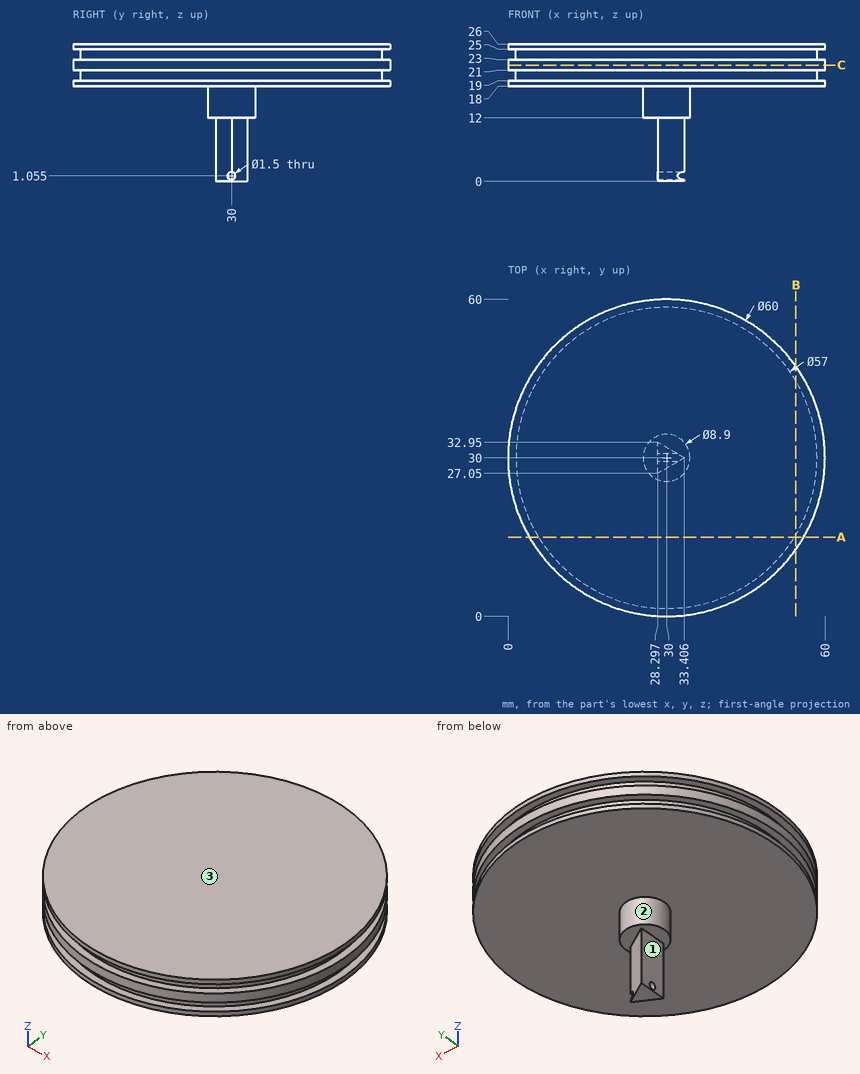
Input: dimensioned drawing with shaded views. Units: mm. Origin: part minimum x, y, z. A direction names the side the tool comes from. Give positions to 0.01 mm unless a question says otherwise; leave off trailing zeros. Order: outer loops, then holes, each group sorted by start corner. A loop starts at its lowest first (then second) coordinate and runs counter-clockwise, first axis right, second up. Notation, with made-up numbers: (62, 19.5) -> (77, 19.5) arc R22 ccw to (77, 31.5) -> close; hole circle Ø9 at (-40, -5.75). An arc over 180 degrees is marked (long way). Use a Markdown table: item, result.
1) Section query C-C, the plane z = 22. Return the cut outline in (x, y).
Answer list:
| item | result |
|---|---|
| outline | circle Ø60 at (30, 30) |
2) Section query A-A, the plane y = 15. Return the cut outline in (x, z).
Answer list:
| item | result |
|---|---|
| outline | (4.02, 18) -> (55.98, 18) -> (55.98, 19) -> (54.23, 19) -> (54.23, 21) -> (55.98, 21) -> (55.98, 23) -> (54.23, 23) -> (54.23, 25) -> (55.98, 25) -> (55.98, 26) -> (4.02, 26) -> (4.02, 25) -> (5.77, 25) -> (5.77, 23) -> (4.02, 23) -> (4.02, 21) -> (5.77, 21) -> (5.77, 19) -> (4.02, 19) -> close |
3) Section query B-B, the plane x = 54.5. Return the cut outline in (y, z), then the cut area to 3 significant figures.
Answer list:
| item | result |
|---|---|
| outline | (12.69, 18) -> (47.31, 18) -> (47.31, 19) -> (44.56, 19) -> (44.56, 21) -> (47.31, 21) -> (47.31, 23) -> (44.56, 23) -> (44.56, 25) -> (47.31, 25) -> (47.31, 26) -> (12.69, 26) -> (12.69, 25) -> (15.44, 25) -> (15.44, 23) -> (12.69, 23) -> (12.69, 21) -> (15.44, 21) -> (15.44, 19) -> (12.69, 19) -> close |
| area | 255 mm² |
4) Ray query, line 1 along Z through (x, y) = (32, 30) (1 decimal); line 2 along Z through (x, y) = (26, 31); line 3 along Z through (x, y) = (39, 11). Return the intervals inside material, ascending. Write a range as [from, to].
Answer list:
| item | result |
|---|---|
| line 1 | [0, 0.3], [1.8, 26] |
| line 2 | [12, 26] |
| line 3 | [18, 26] |
5) Contact query for flat-ended pins moving along their axis: P1, Ø1, axis at y = 7.5, z = 22, coming from the -X side (1 decimal); P2, Ø18, axis at x = 17, y = 20, coming from the -Z side; P3, Ø6.5, axis at y = 30.5, z = 9, coming from the -X side. Output: stop coordinate, or through.
Answer list:
| item | result |
|---|---|
| P1 | x = 9.6 |
| P2 | z = 18 |
| P3 | x = 25.55 |
6) Reachability of the marked faces 1, 2 and 3 from +Z, -Z, +X, -X, +Y, -Y: full face, straight path, thin tool, end or side. Return the list, or none.
Answer list:
| item | result |
|---|---|
| face 1 | -Z, -X, +Y, -Y |
| face 2 | -Z |
| face 3 | +Z, +X, -X, +Y, -Y |
